Verification items for the finished model (mm, model axes). Give positions to 0.01 mm unless a question says otherwise; leave off trailing zeros. Loops run counter-clockwise (first coordinate to the right, second up) from the corner with the lowest first, then second, coordinate; pieces in that order, holes last. Notation, with made-up numbers: (-4, 7) -> (26, 7) arc R7 cw to (26, 17) -> close; hole circle Ø6 at (65.25, 17). An arc over 180 degrees is marked (long way). Answer in a Markdown table with one row per item. Add a question column.
Q1. Section check B-B on x = 0. Enter the section's corners in (y, z).
Q2. Material ranges on probe 1 along X at (y, z) = (0.9, -27); probe 2 along X at (y, z) = (0.5, 7.5); probe 3 along Y at (x, z) = (-2.75, 27), recorded low to high.
Q3. Section check C-C on y = 1.2. Enter the section's corners in (x, z).
Q4. Release check for a two-part mould opening along X. For faces 1 (the face through (12, 1, 0)), 2 (the face through (0.1, 1, -29.5)), 3 (the face through (0, 2, -5)), 4 (the face through (0.751, 1.014, 10.385)) record: pulls with the +X half, pulls with the -X half, needs draft (parallel to the pull), parting line crosses it, or undercut.
Q5. Section check A-A on z = 8. Enter the section's corners in (x, y).
Q6. Gauge pin test, flat ends, axial feed: P1, Ø12, axis at x = 6, z = -12, coming from the -Y side; P2, Ø4.5, axis at x = 0, z = -27, coming from the -Y side. Record the tip position at first contact, or that the pin passes through.
Q7. Section check D-D on z = 29.5. Enter the section's corners in (x, y).
```python
from build123d import *

# Parameters (mm, degrees)
SKETCH_1_W               = 24
SKETCH_1_H               = 70
EXTRUDE_1_DEPTH          = 2
SKETCH_2_R               = 2.5
CUT_EXTRUDE_1_DEPTH      = 38.054014627
CUT_EXTRUDE_2_DEPTH      = 43.485291572
CUT_EXTRUDE_2_DEPTH_BACK = 43.485291572


with BuildPart() as part:
    # 草图1 → 凸台-拉伸1 (new body)
    with BuildSketch(Plane(origin=(0, 0, 0), x_dir=(1, 0, 0), z_dir=(0, 1, 0))):
        Rectangle(SKETCH_1_W, SKETCH_1_H)
    extrude(amount=EXTRUDE_1_DEPTH)

    # 草图2 → 切除-拉伸1 (cut, through all)
    with BuildSketch(Plane(origin=(0, 2, 0), x_dir=(1, 0, 0), z_dir=(0, 1, 0))):
        with Locations(Location((0, -8, 0), (0, 0, 270))):
            Circle(SKETCH_2_R)
        with Locations(Location((0, 27, 0), (0, 0, 270))):
            Circle(SKETCH_2_R)
    extrude(amount=-CUT_EXTRUDE_1_DEPTH, mode=Mode.SUBTRACT)

    # 草图3 → 切除-拉伸2 (cut, two sides: drawn at the far end of the back side and taken through both)
    with BuildSketch(Plane(origin=(12, 0, 0), x_dir=(0, 0, -1), z_dir=(1, 0, 0)).offset(-CUT_EXTRUDE_2_DEPTH_BACK)):
        Polygon((-182.143123104, -29.428624621), (-35, 0), (-25, 2), (122.143123104, 31.428624621), (63.285873863, 325.71487083), (-241.000372346, 264.857621588), align=None)
    extrude(amount=CUT_EXTRUDE_2_DEPTH + CUT_EXTRUDE_2_DEPTH_BACK, mode=Mode.SUBTRACT)


solid = part.part
```
Taken from the geometry:
| question | item | result |
|---|---|---|
| 1 | outline | (0, -35) -> (2, -35) -> (2, -29.5) -> (0, -29.5) -> close; (0, -24.5) -> (2, -24.5) -> (2, 5.5) -> (0, 5.5) -> close; (0, 10.5) -> (2, 10.5) -> (2, 25) -> (0, 35) -> close |
| 2 | probe 1 | x = -12 to -2.5, 2.5 to 12 |
| 2 | probe 2 | x = -12 to -2.45, 2.45 to 12 |
| 2 | probe 3 | y = 0 to 1.6 |
| 3 | outline | (-12, -35) -> (12, -35) -> (12, 29) -> (-12, 29) -> close; hole circle Ø5 at (0, -27); hole circle Ø5 at (0, 8) |
| 4 | face 1 | pulls with the +X half |
| 4 | face 2 | undercut |
| 4 | face 3 | needs draft |
| 4 | face 4 | undercut |
| 5 | outline | (-12, 0) -> (-2.5, 0) -> (-2.5, 2) -> (-12, 2) -> close; (2.5, 0) -> (12, 0) -> (12, 2) -> (2.5, 2) -> close |
| 6 | P1 | stops at y = 0 |
| 6 | P2 | passes through |
| 7 | outline | (-12, 0) -> (12, 0) -> (12, 1.1) -> (-12, 1.1) -> close |
